Can you work these out from the drawing? Everything is in mm from the part's minimum corner. Round coordinates to 2 decimals unless told otherwise and drop trailing zeros. Loops run counter-clockwise (first coordinate to the right, second up) from the corner with the lowest first, then second, coordinate; pieces in that order, holes last. Notation, with made-up numbers: (-26.75, 0) - (1.25, 0) arc R27 ccw to (1.25, 27) - close; hole circle Ø2 at (57.25, -38). An arc over 180 degrees is marked (long way). Return JSON: item names as keys, results as strings. Group by question number.
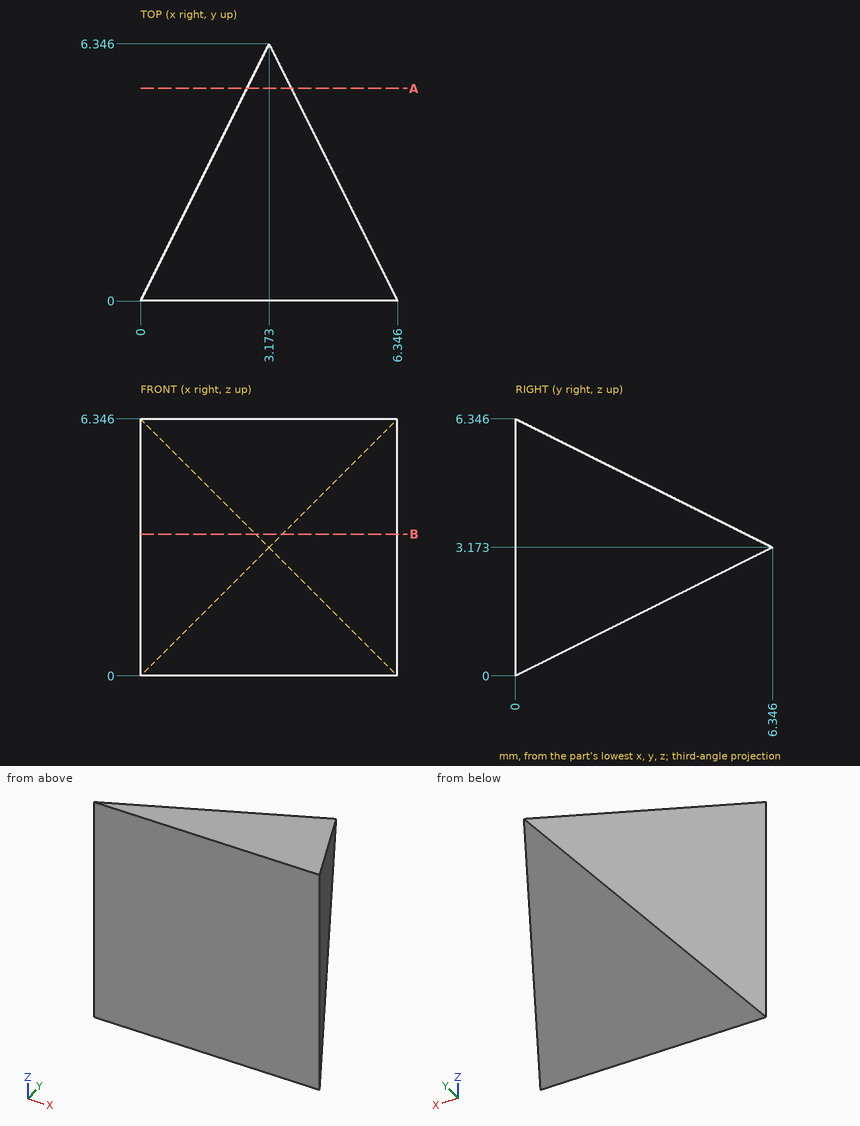
Q1. Imagine slicing it at B-B, the plane z = 3.5. List the corners of the cut face in (x, y) for me (1 decimal).
Q2. Will these pins go through, and if not, where does the flat tip stop? pin 1 Ø3 at (x, y) = (5.5, 4.5) entering from -Z; pin 2 Ø3 at (y, z) = (3, 2) entering from -X; pin 3 Ø1 at (x, z) = (2, 3) entering from +Y.
Q3. Please list where these lines run through material, in increasing order: line 1 (Y direction, x = 2.25, z = 4); line 2 (Y direction, x = 1, z = 6) (1 decimal); line 3 (Z direction, x = 1.25, y = 2) (1 decimal).
Q4. Imagine slicing it at A-A, the plane y = 5.25. List the corners of the cut face in (x, z) for me (1 decimal).
Output values:
{
 "1": {"outline": "(0, 0) - (6.3, 0) - (3.5, 5.7) - (2.8, 5.7) - close"},
 "2": {"pin 1": "stops at z = 1.6", "pin 2": "stops at x = 0.75", "pin 3": "stops at y = 5"},
 "3": {"line 1": "y = 0 to 4.5", "line 2": "y = 0 to 0.7", "line 3": "z = 1 to 5.3"},
 "4": {"outline": "(2.6, 2.6) - (3.7, 2.6) - (3.7, 3.7) - (2.6, 3.7) - close"}
}
